from build123d import *

# Parameters (mm, degrees)
F0_R     = 524.5
F0_R_2   = 5.25
F0_R_3   = 26
F1_DEPTH = 5


with BuildPart() as f1:
    # F0 (on Top) → F1 (new body)
    with BuildSketch(Plane.XY):
        Circle(F0_R)
        with Locations((-205.490317, -149.297454)):
            Circle(F0_R_2, mode=Mode.SUBTRACT)
        with Locations((-78.490317, -241.568355)):
            Circle(F0_R_2, mode=Mode.SUBTRACT)
        with Locations((78.490317, -241.568355)):
            Circle(F0_R_2, mode=Mode.SUBTRACT)
        with Locations((205.490317, -149.297454)):
            Circle(F0_R_2, mode=Mode.SUBTRACT)
        with Locations((-254, 0)):
            Circle(F0_R_2, mode=Mode.SUBTRACT)
        with Locations((-205.490317, 149.297454)):
            Circle(F0_R_2, mode=Mode.SUBTRACT)
        with Locations((-78.490317, 241.568355)):
            Circle(F0_R_2, mode=Mode.SUBTRACT)
        Circle(F0_R_3, mode=Mode.SUBTRACT)
        with Locations((254, 0)):
            Circle(F0_R_2, mode=Mode.SUBTRACT)
        with Locations((78.490317, 241.568355)):
            Circle(F0_R_2, mode=Mode.SUBTRACT)
        with Locations((205.490317, 149.297454)):
            Circle(F0_R_2, mode=Mode.SUBTRACT)
    extrude(amount=F1_DEPTH)


solid = f1.part
Part model, mm, in its own coordinate system. Give positions to 0.01 mm unless a question says otherwise; leave off trailing zeros. Loops run counter-clockwise (first coordinate to the right, second up) from the corner with the lowest first, then second, coordinate; pieces in that order, holes last. Notation, with made-up numbers: M -33,-35 L -27,-35 A25 ccw -27,-10 Z; hole C 5.25,0.25 d4. An arc over 180 degrees is marked long. Put each result on its own line as item: value. Start each with the question number.
1) Saw through at D-D (x = 223). List the corners of the cut face in (y, z).
2) Probe probe 1 along Y at (x, z) = (-10, 3.25); probe 2 along Y at (x, z) = (-254, 2.15); probe 3 along Y at (x, z) = (294, 1.7). List the from-to ranges inside material, lowest first.
3) Flat gauge pins, fed straight in: pin 1 (1.5 mm diameter, centred on x = 68, z = 2.5, fed in from +Y); pin 2 (2 mm diameter, centred on x = -273, z = 4, fed in from +Y). Where does each tip first touch, or does it go through?
4) Saw through at C-C (y = 408.5). List the corners of the cut face in (x, z).
5) Saw through at A-A (x = 0). List the corners of the cut face in (y, z).
6) Saw through at B-B (z = 4.15). State how many separate pieces and enclosed holes the cut face has, then the cut area to 3 significant figures.
Numbers:
1. outline: M -474.73,0 L 474.73,0 L 474.73,5 L -474.73,5 Z
2. probe 1: -524.4 to -24, 24 to 524.4
2. probe 2: -458.89 to -5.25, 5.25 to 458.89
2. probe 3: -434.35 to 434.35
3. pin 1: y = 520.17
3. pin 2: y = 448.46
4. outline: M -328.98,0 L 328.98,0 L 328.98,5 L -328.98,5 Z
5. outline: M -524.5,0 L -26,0 L -26,5 L -524.5,5 Z; M 26,0 L 524.5,0 L 524.5,5 L 26,5 Z
6. separate pieces: 1
6. enclosed holes: 11
6. area: 861,000 mm^2
